Check sheet for the modelled part. Datum: model origin and axes. Units: mm. A direction names the side the tool comes from. Round coordinates to 2 decimals unless told otherwise and drop trailing zeros. Write each loop counter-clockwise with the first axis right and the second up, starting at its lowest first coordinate (ties: lowest second). Pieces come first, ordered by that corner, then holes.
Item 1: Release check for a two-part mould opening along Y. For faces 1 (the flat face through (50, -25, 2)), 2 (the flat face through (-7, -39, 2)), 3 (the flat face through (-4, -4, 2)), 4 (the cylindrical face through (24.08, -25.7, 2.54)) record: pulls with the +Y half, pulls with the -Y half, needs draft (parallel to the pull), parting line crosses it, or undercut.
Item 2: Material ranges on line 1 along Y through (x, z) = (25, 2.4); line 2 along X through (y, z) = (-22, 4.25); line 3 along Y through (x, z) = (24.5, 2.7), recorded low to high.
Item 3: Set-up check for faces 5 (the flat face through (54, -19, 2)), 6 (the flat face through (0, -25, 2)), 7 (the flat face through (54, -46, 2)), 8 (the flat face through (53, -4, 2)): record each of +Z, -Z, +X, -X, +Y, -Y from which the full face is reachable in a straight line by a thin tool's end or side.
Item 4: Section check A-A, the plane y = -25. Record the cut outline in (x, z), plus the area to 3 significant figures.
Item 5: Section check B-B, the plane x = 25. Record the cut outline in (y, z), plus the area to 3 significant figures.
Item 6: Depth check by flat-ended pin: pin 1 (1.2 mm diameter, centred on y = -3, z = 1.5, fed in from -X); pin 2 (1.2 mm diameter, centred on y = -2, z = 2, fed in from +X); pin 3 (2.5 mm diameter, centred on x = 54.5, z = 3, fed in from -Y). Enter the tip coordinate at first touch or a pass-through.
Item 7: Section check C-C, the plane z = 3.45. Record the cut outline in (x, y).
from build123d import *

# Parameters (mm, degrees)
BOSS_EXTRUDE1_DEPTH = 5
SKETCH2_R           = 1.155281189
CUT_EXTRUDE1_DEPTH  = 10


with BuildPart() as part:
    # Sketch1 → Boss-Extrude1 (new body)
    with BuildSketch(Plane.XY):
        Polygon((0, 0), (50, 0), (50, -4), (57, -4), (57, -19), (50, -19), (50, -31), (57, -31), (57, -46), (50, -46), (50, -50), (0, -50), (0, -46), (-7, -46), (-7, -31), (0, -31), (0, -19), (-7, -19), (-7, -4), (0, -4), align=None)
    extrude(amount=BOSS_EXTRUDE1_DEPTH)

    # Sketch2 → Cut-Extrude1 (cut)
    with BuildSketch(Plane.XY.offset(5)):
        with Locations((25, -25)):
            Circle(SKETCH2_R)
    extrude(amount=-CUT_EXTRUDE1_DEPTH, mode=Mode.SUBTRACT)


solid = part.part
Values found:
1. face 1: undercut
1. face 2: needs draft
1. face 3: pulls with the +Y half
1. face 4: undercut
2. line 1: y = -50 to -26.16, -23.84 to 0
2. line 2: x = 0 to 50
2. line 3: y = -50 to -26.04, -23.96 to 0
3. face 5: +Z, -Z, +X
3. face 6: +Z, -Z, -X
3. face 7: +Z, -Z, +X, -Y
3. face 8: +Z, -Z, +X, +Y
4. outline: (0, 0) - (23.84, 0) - (23.84, 5) - (0, 5) - close; (26.16, 0) - (50, 0) - (50, 5) - (26.16, 5) - close
4. area: 238 mm2
5. outline: (-50, 0) - (-26.16, 0) - (-26.16, 5) - (-50, 5) - close; (-23.84, 0) - (0, 0) - (0, 5) - (-23.84, 5) - close
5. area: 238 mm2
6. pin 1: stops at x = 0
6. pin 2: stops at x = 50
6. pin 3: stops at y = -46
7. outline: (-7, -46) - (0, -46) - (0, -50) - (50, -50) - (50, -46) - (57, -46) - (57, -31) - (50, -31) - (50, -19) - (57, -19) - (57, -4) - (50, -4) - (50, 0) - (0, 0) - (0, -4) - (-7, -4) - (-7, -19) - (0, -19) - (0, -31) - (-7, -31) - close; hole circle Ø2.31 at (25, -25)
